Work out the finished part from the listing and answer in its coordinate system (mm). Face numbers are marked on the shaded views. A direction names the side the tool comes from. Round coordinates to 2 decimals unless told otherwise and drop trailing zeros. Order: outer loops, then holes, each group sorted by start corner. A loop starts at its lowest first (then second) coordinate and runs counter-clockwise, first axis right, second up. Notation, with made-up numbers: (73.25, 59.25) - (121.25, 59.25) arc R16 ccw to (121.25, 79.25) - close; hole circle Ø5 at (-34.75, 82). An arc over 180 degrees is marked (long way). One line per question, with ' | ' between items. Start each with the question number.
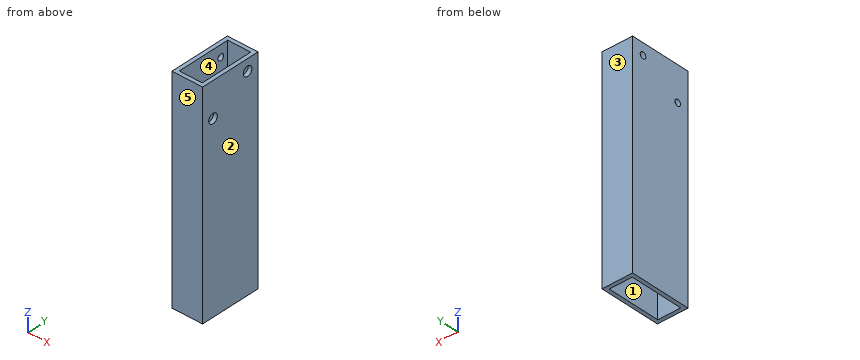
from build123d import *

# Parameters (mm, degrees)
SKETCH1_W           = 25.4
SKETCH1_H           = 50.8
SKETCH1_W_2         = 19.05
SKETCH1_H_2         = 44.45
BOSS_EXTRUDE1_DEPTH = 177.8
SKETCH2_R           = 2.5796875
CUT_EXTRUDE1_DEPTH  = 182.392282085
CUT_EXTRUDE2_REACH  = 183.392
SKETCH3_R           = 3.937


with BuildPart() as part:
    # Sketch1 → Boss-Extrude1 (new body)
    with BuildSketch(Plane.XY):
        Rectangle(SKETCH1_W, SKETCH1_H)
        Rectangle(SKETCH1_W_2, SKETCH1_H_2, mode=Mode.SUBTRACT)
    extrude(amount=BOSS_EXTRUDE1_DEPTH)

    # Sketch2 → Cut-Extrude1 (cut, through all)
    with BuildSketch(Plane(origin=(12.7, 0, 0), x_dir=(0, 0, -1), z_dir=(1, 0, 0))):
        with Locations((-168.275, 15.875)):
            Circle(SKETCH2_R)
        with Locations((-149.225, -15.875)):
            Circle(SKETCH2_R)
    extrude(amount=-CUT_EXTRUDE1_DEPTH, mode=Mode.SUBTRACT)

    # Sketch3 → Cut-Extrude2 (cut, up to next)
    with BuildSketch(Plane(origin=(12.7, 0, 0), x_dir=(0, 0, -1), z_dir=(1, 0, 0)), mode=Mode.PRIVATE) as cut_extrude2_sk1:
        with Locations((-168.275, 15.875)):
            Circle(SKETCH3_R)
    cut_extrude2_tool1 = extrude(cut_extrude2_sk1.sketch, amount=-CUT_EXTRUDE2_REACH, mode=Mode.PRIVATE) & part.part
    # Sketch3 → Cut-Extrude2 (cut, up to next)
    with BuildSketch(Plane(origin=(12.7, 0, 0), x_dir=(0, 0, -1), z_dir=(1, 0, 0)), mode=Mode.PRIVATE) as cut_extrude2_sk2:
        with Locations((-149.225, -15.875)):
            Circle(SKETCH3_R)
    cut_extrude2_tool2 = extrude(cut_extrude2_sk2.sketch, amount=-CUT_EXTRUDE2_REACH, mode=Mode.PRIVATE) & part.part
    add(cut_extrude2_tool1.solids().sort_by_distance((12.7, 15.875, 168.275))[0], mode=Mode.SUBTRACT)
    add(cut_extrude2_tool2.solids().sort_by_distance((12.7, -15.875, 149.225))[0], mode=Mode.SUBTRACT)


solid = part.part
1) Section B-B on x = -7.5 is taken. Give the vertices of the cut face in (y, z) (3 decimals), and give its area (3 significant figures).
2) Determine the mould class of the marked faces 1, 2 and 3 for opening direction Y: released by +Y, released by -Y, zero draft, split by the parting line, or undercut.
3) Section A-A on y = 6 is taken. Give the vertices of the cut face in (x, z) (3 decimals), and give its area (3 significant figures).
4) Section C-C on z = 88 is taken. Give the vertices of the cut face in (x, y) (3 decimals), and give its area (3 significant figures).
5) For the marked faces 4 and 5, determine the directions among +Z, -Z, +X, -X, +Y, -Y from which every point of the face is accessible in a straight line to the end or side of a thin tool.
6) Straight lines are drawn through the part: line 1 (Y direction, x = -8.75, z = 12.5) (3 decimals); line 2 (X direction, y = -10.5, z = 170.5) (3 decimals); line 3 (Z direction, x = 10.5, y = 15.5). For each, find the intervals that lie inside material, in ascending order.
Recorded:
1) outline: (-25.4, 0) - (-22.225, 0) - (-22.225, 177.8) - (-25.4, 177.8) - close; (22.225, 0) - (25.4, 0) - (25.4, 177.8) - (22.225, 177.8) - close | area: 1,130 mm²
2) face 1: undercut | face 2: zero draft | face 3: released by +Y
3) outline: (-12.7, 0) - (-9.525, 0) - (-9.525, 177.8) - (-12.7, 177.8) - close; (9.525, 0) - (12.7, 0) - (12.7, 177.8) - (9.525, 177.8) - close | area: 1,130 mm²
4) outline: (-12.7, -25.4) - (12.7, -25.4) - (12.7, 25.4) - (-12.7, 25.4) - close; hole (-9.525, -22.225) - (9.525, -22.225) - (9.525, 22.225) - (-9.525, 22.225) - close | area: 444 mm²
5) face 4: +Z, -Z | face 5: +Z, -Z, +X, -X, -Y
6) line 1: y = -25.4 to -22.225, 22.225 to 25.4 | line 2: x = -12.7 to -9.525, 9.525 to 12.7 | line 3: z = 0 to 164.36, 172.19 to 177.8
